Build history of the part. All positions in model axes, mm. Face numbers are marked on the shaded views. A direction names the side the tool comes from. Round coordinates to 2 decimals unless told otherwise and drop trailing zeros. Write each loop counter-clockwise with the first axis right and the second up, starting at its lowest first coordinate (ties: lowest second). Pieces come first, ordered by that corner, then holes. Notation, with made-up numbers: M 57.25,-30.5 L 93.25,-30.5 A22 cw 93.25,-16.5 Z; hole C 72.5,8.5 d1. An arc over 180 degrees is marked long. Write item = value, one per line.
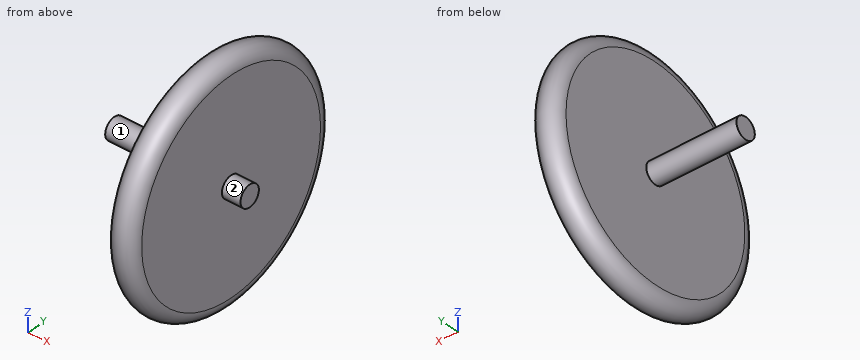
from build123d import *


with BuildPart() as part:
    # Esquisse1 → Révolution1 (revolve)
    with BuildSketch(Plane.XY):
        with BuildLine():
            Line((-2.5, 19.5), (-2.5, 2))
            Line((-2.5, 2), (-19.5, 2))
            Line((-19.5, 2), (-19.5, 0))
            Line((-19.5, 0), (0, 0))
            Line((0, 0), (6, 0))
            Line((6, 0), (6, 2))
            Line((6, 2), (2.5, 2))
            Line((2.5, 2), (2.5, 19.5))
            ThreePointArc((2.5, 19.5), (0, 22), (-2.5, 19.5))
        make_face()
    revolve(axis=Axis((0, 0, 0), (-1, 0, 0)))


solid = part.part
1. Probe probe 1 along X at (y, z) = (8, 7.5); probe 2 along Y at (x, z) = (0.25, 10); probe 3 along Y at (x, z) = (-3.25, -1.5). List the from-to ranges inside material, lowest first.
Responses:
probe_1 = -2.5 to 2.5
probe_2 = -19.58 to 19.58
probe_3 = -1.32 to 1.32
2. Tool access for the marked faces 1 and 2: list every direction of +Z, -Z, +X, -X, +Y, -Y with a clear straight run to the whole face (end or side of a thin tool).
Responses:
face_1 = -X
face_2 = +X
3. Band-saw the part on C-C (x = -9.75). List the corners of the cut face in (y, z), plus the area to 3 significant figures.
Responses:
outline = C 0,0 d4
area = 12.6 mm²
4. Band-saw the part on A-A (y = 0). List the corners of the cut face in (x, z), plus the area to 3 significant figures.
Responses:
outline = M -19.5,-2 L -2.5,-2 L -2.5,-19.5 A2.5 ccw 2.5,-19.5 L 2.5,-2 L 6,-2 L 6,2 L 2.5,2 L 2.5,19.5 A2.5 ccw -2.5,19.5 L -2.5,2 L -19.5,2 Z
area = 297 mm²
5. Flat gauge pins, fed straight in: pin 1 (1 mm diameter, centred on x = -9.5, y = 4, fed in from +Z); pin 2 (8 mm diameter, centred on x = -11, y = -5, fed in from -Z); pin 3 (6 mm diameter, centred on y = -4, z = 16, fed in from +X); pin 4 (10 mm diameter, centred on x = 2, y = 2, fed in from +Z). Where does each tip first touch, or does it go through?
Responses:
pin_1 = through
pin_2 = -1.73
pin_3 = 2.5
pin_4 = 22
